```python
from build123d import *

# Parameters (mm, degrees)
F1_DEPTH = 30
F3_D     = 3.4
F5_DEPTH = 25
F6_D     = 6.6


# Not quite as in the source:
# - a feature names something its author has since deleted; it is built from what else it names


with BuildPart() as f1:
    # F0 (on Right) → F1 (new body)
    with BuildSketch(Plane.YZ):
        Polygon((0, 60), (0, 0), (40.3389412612, 0), (40.3389412612, 8), (8.3389412612, 8), (8.3389412612, 60), align=None)
    extrude(amount=F1_DEPTH)

    # F3 (through all)
    with Locations(Plane.XZ):
        with Locations((4, 56), (4, 18)):
            Hole(F3_D / 2)

    # F4 (on face) → F5 (cut)
    with BuildSketch(Plane(origin=(0, 0, 0), x_dir=(1, 0, 0), z_dir=(0, 0, -1))):
        with BuildLine():
            ThreePointArc((8.2706560702, -26.1462763052), (7.66, -25.9585094241), (7.0246071276, -25.8919276299))
            ThreePointArc((7.0246071276, -25.8919276299), (7.6465318102, -26.0244898096), (8.2706560702, -26.1462763052))
        make_face()
        with BuildLine():
            ThreePointArc((22.9753928724, -25.8919276299), (22.34, -25.9585094241), (21.7293439298, -26.1462763052))
            ThreePointArc((21.7293439298, -26.1462763052), (22.3534681898, -26.0244898096), (22.9753928724, -25.8919276299))
        make_face()
        with BuildLine():
            ThreePointArc((19.7422005642, -29.7178994133), (15, -30), (10.2577994358, -29.7178994133))
            ThreePointArc((10.2577994358, -29.7178994133), (8.9379952514, -31.8628234183), (6.4894588415, -32.4521039296))
            ThreePointArc((6.4894588415, -32.4521039296), (15, -33.2967716909), (23.5105411585, -32.4521039296))
            ThreePointArc((23.5105411585, -32.4521039296), (21.0620047486, -31.8628234183), (19.7422005642, -29.7178994133))
        make_face()
        with BuildLine():
            ThreePointArc((10.3, -29.1918358845), (10.2894329403, -29.455712619), (10.2577994358, -29.7178994133))
            ThreePointArc((10.2577994358, -29.7178994133), (15, -30), (19.7422005642, -29.7178994133))
            ThreePointArc((19.7422005642, -29.7178994133), (20.1162784073, -27.5874201728), (21.7293439298, -26.1462763052))
            ThreePointArc((21.7293439298, -26.1462763052), (15, -26.767340949), (8.2706560702, -26.1462763052))
            ThreePointArc((8.2706560702, -26.1462763052), (9.7461941876, -27.3619677242), (10.3, -29.1918358845))
        make_face()
        with BuildLine():
            ThreePointArc((7.0246071276, -25.8919276299), (4.9757761074, -26.5855899958), (3.7966505642, -28.3990229227))
            ThreePointArc((3.7966505642, -28.3990229227), (7, -29.1918358845), (10.2577994358, -29.7178994133))
            ThreePointArc((10.2577994358, -29.7178994133), (10.2894329403, -29.455712619), (10.3, -29.1918358845))
            ThreePointArc((10.3, -29.1918358845), (9.7461941876, -27.3619677242), (8.2706560702, -26.1462763052))
            ThreePointArc((8.2706560702, -26.1462763052), (7.6465318102, -26.0244898096), (7.0246071276, -25.8919276299))
        make_face()
        with BuildLine():
            ThreePointArc((10.2577994358, -29.7178994133), (7, -29.1918358845), (3.7966505642, -28.3990229227))
            ThreePointArc((3.7966505642, -28.3990229227), (4.170235318, -30.8896084972), (6.1919389643, -32.3913729389))
            ThreePointArc((6.1919389643, -32.3913729389), (6.3406456618, -32.421999261), (6.4894588415, -32.4521039296))
            ThreePointArc((6.4894588415, -32.4521039296), (8.9379952514, -31.8628234183), (10.2577994358, -29.7178994133))
        make_face()
        with BuildLine():
            ThreePointArc((26.2033494358, -28.3990229227), (23, -29.1918358845), (19.7422005642, -29.7178994133))
            ThreePointArc((19.7422005642, -29.7178994133), (21.0620047486, -31.8628234183), (23.5105411585, -32.4521039296))
            ThreePointArc((23.5105411585, -32.4521039296), (23.6593543382, -32.421999261), (23.8080610357, -32.3913729389))
            ThreePointArc((23.8080610357, -32.3913729389), (25.6035169884, -31.2195684337), (26.3, -29.1918358845))
            ThreePointArc((26.3, -29.1918358845), (26.2757482457, -28.7924946382), (26.2033494358, -28.3990229227))
        make_face()
        with BuildLine():
            ThreePointArc((21.7293439298, -26.1462763052), (20.1162784073, -27.5874201728), (19.7422005642, -29.7178994133))
            ThreePointArc((19.7422005642, -29.7178994133), (23, -29.1918358845), (26.2033494358, -28.3990229227))
            ThreePointArc((26.2033494358, -28.3990229227), (25.0242238926, -26.5855899958), (22.9753928724, -25.8919276299))
            ThreePointArc((22.9753928724, -25.8919276299), (22.3534681898, -26.0244898096), (21.7293439298, -26.1462763052))
        make_face()
    extrude(amount=-F5_DEPTH, mode=Mode.SUBTRACT)

    # F6 (through all)
    with Locations(Plane(origin=(0, 0, 0), x_dir=(1, 0, 0), z_dir=(0, 0, -1))):
        with Locations((15, -15)):
            Hole(F6_D / 2)


solid = f1.part
```
Build history of the part. All positions in model axes, mm. A direction names the side the tool comes from. Coordinates: 2 decimals unless noted, no trailing zeros. Write each loop counter-clockwise with the first axis right and the second up, starting at its lowest first coordinate (ties: lowest second). Pieces come first, ordered by that corner, then holes.
1. Band-saw the part on C-C, the plane x = 15. Give the cut face in (y, z).
Answer block:
outline: (0, 0) - (11.7, 0) - (11.7, 8) - (8.34, 8) - (8.34, 60) - (0, 60) - close; (18.3, 0) - (26.77, 0) - (26.77, 8) - (18.3, 8) - close; (33.3, 0) - (40.34, 0) - (40.34, 8) - (33.3, 8) - close
2. Band-saw the part on A-A, the plane y = 15. Give the cut face in (x, z), and give its area (3 significant figures).
Answer block:
outline: (0, 0) - (11.7, 0) - (11.7, 8) - (0, 8) - close; (18.3, 0) - (30, 0) - (30, 8) - (18.3, 8) - close
area: 187 mm2
3. 3-axis set-ups, long thin cutter, end or side, ignore diameter. For faces 1 (the flat face through (15, 8.339, 34)), 2 (the flat face through (15, 0, 30)), 3 (the cylindrical face through (15.095, 26.767, 3.944)): which of +Z, -Z, +X, -X, +Y, -Y reach the whole face in a straight line?
Answer block:
face 1: +Z, +X, -X, +Y
face 2: +Z, -Z, +X, -X, -Y
face 3: +Z, -Z
4. Pull direction X, two halves, no side cores. Call faces 4 (the cylindrical face through (18.3, 14.9, 4.1)), 5 (the flat face through (0, 8, 23)), 6 (the cylindrical face through (3.086, 4.228, 19.433)), 7 (the flat face through (15, 20, 0)): released by +X, released by -X, zero draft, split by the parting line, or undercut.
Answer block:
face 4: undercut
face 5: released by -X
face 6: undercut
face 7: zero draft
5. Band-saw the part on B-B, the plane z = 56. Give the cut face in (x, y).
Answer block:
outline: (0, 0) - (2.3, 0) - (2.3, 8.34) - (0, 8.34) - close; (5.7, 0) - (30, 0) - (30, 8.34) - (5.7, 8.34) - close
6. Drill centre lines: probe 1 along Z at (x, y) = (4, 3); probe 2 along X at (y, z) = (15, 4); probe 3 along Z at (x, y) = (10.5, 35). Where is each one in solid material? Low to high.
Answer block:
probe 1: z = 0 to 16.3, 19.7 to 54.3, 57.7 to 60
probe 2: x = 0 to 11.7, 18.3 to 30
probe 3: z = 0 to 8
7. Drop flat-ended pins along their axis: pin 1 (1 mm diameter, centred on x = 25, y = 31, fed in from -Z); pin 2 (1.5 mm diameter, centred on x = 12.5, z = 24, fed in from -Y); pin 3 (6 mm diameter, centred on x = 16.5, y = 30.5, fed in from +Z). Give the stop position or say it passes through.
Answer block:
pin 1: passes through
pin 2: stops at y = 0
pin 3: stops at z = 8
8. Band-saw the part on D-D, the plane z = 7. Give the cut face in (x, y).
Answer block:
outline: (0, 0) - (30, 0) - (30, 40.34) - (0, 40.34) - close; hole (6.19, 32.39) arc R3.3 ccw (long way) to (8.27, 26.15) arc R36.77 cw to (21.73, 26.15) arc R3.3 ccw (long way) to (23.81, 32.39) arc R43.3 ccw to (23.51, 32.45) arc R43.3 ccw to (6.49, 32.45) arc R43.3 ccw to start; hole circle Ø6.6 at (15, 15)
